```python
from build123d import *

# Parameters (mm, degrees)
SKETCH_1_R                  = 5
EXTRUDE_1_DEPTH             = 10.5
EXTRUDE_1_DEPTH_BACK        = 10.5
EXTRUDE_3_DEPTH             = 4.5
EXTRUDE_3_DEPTH_BACK        = 4.5
SKETCH_7_R                  = 6
EXTRUDE_4_DEPTH             = 3
SKETCH_8_R                  = 6
EXTRUDE_5_DEPTH             = 3
SKETCH_9_R                  = 9.5
CUT_EXTRUDE_1_DEPTH         = 7
SKETCH_10_R                 = 8.5
CUT_EXTRUDE_2_DEPTH         = 9
HOLE_WIZARD_M4_1_D          = 3.3
SKETCH_22_W                 = 46.630089335
SKETCH_22_H                 = 20.014444788
CUT_EXTRUDE_3_DEPTH         = 1111
HOLE_WIZARD_M3_2_D          = 2.5
PATTERN_LINEAR_1_COUNT      = 3
PATTERN_LINEAR_1_PITCH      = 70
PATTERN_LINEAR_1_COUNT_DIR2 = 2
PATTERN_LINEAR_1_PITCH_DIR2 = 10
HOLE_WIZARD_M3_1_D          = 2.5
PATTERN_CIRCULAR_1_COUNT    = 6
SKETCH_32_R                 = 1.25
EXTRUDE_6_DEPTH             = 3.5


with BuildPart() as part:
    # Sketch 1 → Extrude 1 (new body, two sides)
    with BuildSketch(Plane(origin=(0, 0, 0), x_dir=(1, 0, 0), z_dir=(0, 1, 0))) as extrude_1_sk:
        Circle(SKETCH_1_R)
    extrude(amount=EXTRUDE_1_DEPTH)
    extrude(extrude_1_sk.sketch, amount=-EXTRUDE_1_DEPTH_BACK)

    # Sketch 6 → Extrude 3 (add, two sides)
    with BuildSketch(Plane(origin=(0, 0, 0), x_dir=(1, 0, 0), z_dir=(0, 1, 0))) as extrude_3_sk:
        with BuildLine():
            Line((-12.5, 0), (-12.5, -260))
            ThreePointArc((-12.5, -260), (0, -272.5), (12.5, -260))
            Line((12.5, -260), (12.5, 0))
            ThreePointArc((12.5, 0), (0, 12.5), (-12.5, 0))
        make_face()
    extrude(amount=EXTRUDE_3_DEPTH)
    extrude(extrude_3_sk.sketch, amount=-EXTRUDE_3_DEPTH_BACK)

    # Sketch 7 → Extrude 4 (add)
    with BuildSketch(Plane.XZ.offset(4.5)):
        Circle(SKETCH_7_R)
    extrude(amount=EXTRUDE_4_DEPTH)

    # Sketch 8 → Extrude 5 (add)
    with BuildSketch(Plane(origin=(0, 4.5, 0), x_dir=(1, 0, 0), z_dir=(0, 1, 0))):
        Circle(SKETCH_8_R)
    extrude(amount=EXTRUDE_5_DEPTH)

    # Sketch 9 → Cut-Extrude 1 (cut)
    with BuildSketch(Plane.XZ.offset(4.5)):
        with Locations((0, 250)):
            Circle(SKETCH_9_R)
    extrude(amount=-CUT_EXTRUDE_1_DEPTH, mode=Mode.SUBTRACT)

    # Sketch 10 → Cut-Extrude 2 (cut, through all)
    with BuildSketch(Plane.XZ.offset(-2.5)):
        with Locations((0, 250)):
            Circle(SKETCH_10_R)
    extrude(amount=-CUT_EXTRUDE_2_DEPTH, mode=Mode.SUBTRACT)

    # Hole Wizard M4 _ _ _ _1 (through all)
    with Locations(Plane(origin=(0, -10.5, 0), x_dir=(-1, 0, 0), z_dir=(0, -1, 0))):
        with Locations((0, 0)):
            Hole(HOLE_WIZARD_M4_1_D / 2)

    # Sketch 22 → Cut-Extrude 3 (cut, symmetric)
    with BuildSketch(Plane.XY):
        with Locations((-0.058287612, -9.007222394)):
            Rectangle(SKETCH_22_W, SKETCH_22_H)
    extrude(amount=CUT_EXTRUDE_3_DEPTH, both=True, mode=Mode.SUBTRACT)

    # Hole Wizard M3 _ _ _ _2 (through all)
    with Locations(Plane(origin=(0, 1, 0), x_dir=(-1, 0, 0), z_dir=(0, -1, 0))):
        with Locations((5, -15)):
            hole_wizard_m3_2 = Hole(HOLE_WIZARD_M3_2_D / 2)

    # Pattern Linear 1: Hole Wizard M3 _ _ _ _2 3 × 2
    with Locations(*[(j * PATTERN_LINEAR_1_PITCH_DIR2, 0, i * PATTERN_LINEAR_1_PITCH) for i in range(PATTERN_LINEAR_1_COUNT) for j in range(PATTERN_LINEAR_1_COUNT_DIR2) if (i, j) != (0, 0)]):
        add(hole_wizard_m3_2, mode=Mode.SUBTRACT)

    # Hole Wizard M3 _ _ _ _1 (through all)
    with Locations(Plane(origin=(0, 1, 0), x_dir=(-1, 0, 0), z_dir=(0, -1, 0))):
        with Locations((6.75, -261.691342951)):
            hole_wizard_m3_1 = Hole(HOLE_WIZARD_M3_1_D / 2)

    # Pattern Circular 1: Hole Wizard M3 _ _ _ _1 ×6 about axis, 2 skipped
    pattern_circular_1_axis = Axis((0, 2.5, 250), (0, -1, 0))
    add([hole_wizard_m3_1.rotate(pattern_circular_1_axis, i * 360 / PATTERN_CIRCULAR_1_COUNT) for i in range(1, PATTERN_CIRCULAR_1_COUNT) if i not in (1, 4)], mode=Mode.SUBTRACT)

    # Sketch 32 → Extrude 6 (add)
    with BuildSketch(Plane.XZ.offset(-1)):
        with Locations((-5, 15)):
            Circle(SKETCH_32_R)
        with Locations((5, 15)):
            Circle(SKETCH_32_R)
    extrude(amount=-EXTRUDE_6_DEPTH)


solid = part.part
```
Verification items for the finished model (mm, model axes). A direction names the side the tool comes from. Coordinates: 2 decimals unless noted, no trailing zeros. Loops run counter-clockwise (first coordinate to the right, second up) from the corner with the lowest first, then second, coordinate; pieces in that order, holes last. Notation, with made-up numbers: (63, 74) -> (76, 74) arc R19 cw to (76, 105) -> close; hole circle Ø7 at (-14, 54). An arc over 180 degrees is marked (long way). Answer in a Markdown table with one row per item.
1) Scan lines: line 1 along X through (y, z) = (3.5, 155); line 2 along Z through (x, y) = (-5, 3.5); line 3 along Y through (x, z) = (-6.25, 89.5). Record each from-to range of solid material in increasing order. Write a range as from..to.
The answers:
| item | result |
|---|---|
| line 1 | x = -12.5..-6.25, -3.75..3.75, 6.25..12.5 |
| line 2 | z = -11.46..83.75, 86.25..153.75, 156.25..243.13, 256.87..271.46 |
| line 3 | y = 1..4.5 |
2) Access from +Z, -Z, +X, -X, +Y, -Y to the whole of each face (thin tool, end or side, straight path). Record for faces 5 (the face through (-2.059, 1.739, 240.726)), 6 (the face through (2, 10.5, 0)), 7 (the face through (-6, 6, 0)).
The answers:
| item | result |
|---|---|
| face 5 | -Y |
| face 6 | +Z, -Z, +X, -X, +Y |
| face 7 | +Y |
3) Draft check along Z on faces 1 (the face through (-1.107, 3.486, 258.428)), 2 (the face through (-2.2, 2.5, 241.6)), 3 (the face through (0.275, 2.774, -12.497)), 4 (the face through (-1.08, 9.02, 4.88)). Enter one of: released by +Z, released by -Z, zero draft, split by the parting line, or undercut.
The answers:
| item | result |
|---|---|
| face 1 | undercut |
| face 2 | undercut |
| face 3 | released by -Z |
| face 4 | split by the parting line |
4) Section check B-B (z = 203.5). Record the cut outline in (x, y).
The answers:
| item | result |
|---|---|
| outline | (-12.5, 1) -> (12.5, 1) -> (12.5, 4.5) -> (-12.5, 4.5) -> close |
5) Depth check by flat-ended pin: P1, Ø6, axis at x = -0.5, z = 92.5, coming from the +Y side; P2, Ø4, axis at x = 0, z = 0, coming from the -Y side; P3, Ø1, axis at x = -6, y = 4, coming from the -Z side (3 decimals). Enter the tip coordinate at first touch or a pass-through.
The answers:
| item | result |
|---|---|
| P1 | stops at y = 4.5 |
| P2 | stops at y = 1 |
| P3 | stops at z = -11.225 |
6) Section check A-A (z = 250). Record the cut outline in (x, y), and give its area (3 significant figures).
The answers:
| item | result |
|---|---|
| outline | (-12.5, 1) -> (-9.5, 1) -> (-9.5, 2.5) -> (-8.5, 2.5) -> (-8.5, 4.5) -> (-12.5, 4.5) -> close; (8.5, 2.5) -> (9.5, 2.5) -> (9.5, 1) -> (12.5, 1) -> (12.5, 4.5) -> (8.5, 4.5) -> close |
| area | 25.0 mm2 |
